Here's how the part is built. I have some questions about the finished solid (model axes, mm). Face numbers are marked on the shaded views. Coordinates: 2 decimals unless noted, no trailing zeros. Write each loop counter-clockwise with the first axis right and the second up, starting at its lowest first coordinate (ties: lowest second). Pieces come first, ordered by that corner, then holes. Notation, with made-up numbers: (75.5, 56) -> (96.5, 56) arc R14 cw to (96.5, 66) -> close; hole circle Ø7 at (44, 85). An arc over 180 degrees is marked (long way). Use a Markdown table: item, result. Add a question column.
Item 1: Imagine slicing it at A-A, the plane z = 2.85. Write out the boundary of the cut face in (x, y), and give its area (3 significant figures).
Item 2: Will these pins go through, and if not, where does the flat tip stop? pin 1 Ø1.5 at (y, z) = (-13, 1.5) entering from -X; pin 2 Ø1 at (x, y) = (10, -16.5) entering from +Z.
Item 3: If we mould it in two halves opening along Y, with no side actions, what happens to the marked faces 1 and 2? For each: pulls with the +Y half, pulls with the -Y half, needs draft (parallel to the pull), parting line crosses it, or undercut.
Item 4: If I drill on line 1 along Y through (x, z) = (0, 0.45); line 2 along Y through (x, z) = (0.5, 2.1); line 3 along X through (y, z) = (-7, 4.2), over which ranges is the centre line in solid material (lowest first)? Write a range as from..to.
```python
from build123d import *
from OCP.BRepFilletAPI import BRepFilletAPI_MakeChamfer

# Parameters (mm, degrees)
SKETCH_1_R          = 22
SKETCH_1_R_2        = 17.5
EXTRUDE_1_DEPTH     = 5
SKETCH_2_R          = 20.5
SKETCH_2_R_2        = 19
CUT_EXTRUDE_1_DEPTH = 0.5
CHAMFER_1_SIZE      = 0.2
CHAMFER_1_SIZE2     = 0.238350719
CHAMFER_2_SIZE      = 0.2
CHAMFER_2_SIZE2     = 0.238350719


with BuildPart() as part:
    # 草图1 → 凸台-拉伸1 (new body)
    with BuildSketch(Plane.XY):
        Circle(SKETCH_1_R)
        Circle(SKETCH_1_R_2, mode=Mode.SUBTRACT)
    extrude(amount=EXTRUDE_1_DEPTH)

    # 草图2 → 切除-拉伸1 (cut)
    with BuildSketch(Plane.XY.offset(5)):
        Circle(SKETCH_2_R)
        Circle(SKETCH_2_R_2, mode=Mode.SUBTRACT)
    cut_extrude_1 = extrude(amount=-CUT_EXTRUDE_1_DEPTH, mode=Mode.SUBTRACT)

    # 倒角1: one chamfer whose edges measure the first distance from different faces: ONE call of the kernel's chamfer builder (chamfer() names one face for all edges)
    chamfer_1_edges_1 = [part.edges().sort_by_distance(p)[0] for p in [
        (-20.5, 0, 4.5),
    ]]
    chamfer_1_side_1 = [part.faces().sort_by_distance(p)[0] for p in [
        (-20.5, 0, 4.75),
    ]]
    chamfer_1_edges_2 = [part.edges().sort_by_distance(p)[0] for p in [
        (-19, 0, 5),
    ]]
    chamfer_1_side_2 = [part.faces().sort_by_distance(p)[0] for p in [
        (-19, 0, 4.75),
    ]]
    chamfer_1_edges_3 = [part.edges().sort_by_distance(p)[0] for p in [
        (-22, 0, 5),
    ]]
    chamfer_1_side_3 = [part.faces().sort_by_distance(p)[0] for p in [
        (-22, 0, 2.5),
    ]]
    chamfer_1_edges_4 = [part.edges().sort_by_distance(p)[0] for p in [
        (-17.5, 0, 5),
    ]]
    chamfer_1_side_4 = [part.faces().sort_by_distance(p)[0] for p in [
        (-18.462598846, 0, 5),
    ]]
    chamfer_1 = BRepFilletAPI_MakeChamfer(part.part.solid().wrapped)
    for e in chamfer_1_edges_1:
        chamfer_1.Add(CHAMFER_1_SIZE, CHAMFER_1_SIZE2, e.wrapped, chamfer_1_side_1[0].wrapped)  # the first distance lies on this face
    for e in chamfer_1_edges_2:
        chamfer_1.Add(CHAMFER_1_SIZE, CHAMFER_1_SIZE2, e.wrapped, chamfer_1_side_2[0].wrapped)  # the first distance lies on this face
    for e in chamfer_1_edges_3:
        chamfer_1.Add(CHAMFER_1_SIZE, CHAMFER_1_SIZE2, e.wrapped, chamfer_1_side_3[0].wrapped)  # the first distance lies on this face
    for e in chamfer_1_edges_4:
        chamfer_1.Add(CHAMFER_1_SIZE, CHAMFER_1_SIZE2, e.wrapped, chamfer_1_side_4[0].wrapped)  # the first distance lies on this face
    add(Compound.cast(chamfer_1.Shape()), mode=Mode.REPLACE)

    # 镜向1: 切除-拉伸1 across plane
    add(cut_extrude_1.mirror(Plane.XY.offset(2.5)), mode=Mode.SUBTRACT)

    # 倒角2: one chamfer whose edges measure the first distance from different faces: ONE call of the kernel's chamfer builder (chamfer() names one face for all edges)
    chamfer_2_edges_1 = [part.edges().sort_by_distance(p)[0] for p in [
        (-22, 0, 0),
    ]]
    chamfer_2_side_1 = [part.faces().sort_by_distance(p)[0] for p in [
        (-21.377746033, 0, 0),
    ]]
    chamfer_2_edges_2 = [part.edges().sort_by_distance(p)[0] for p in [
        (-19, 0, 0),
    ]]
    chamfer_2_side_2 = [part.faces().sort_by_distance(p)[0] for p in [
        (-18.462598846, 0, 0),
    ]]
    chamfer_2_edges_3 = [part.edges().sort_by_distance(p)[0] for p in [
        (-20.5, 0, 0),
    ]]
    chamfer_2_side_3 = [part.faces().sort_by_distance(p)[0] for p in [
        (-20.5, 0, 0.25),
    ]]
    chamfer_2_edges_4 = [part.edges().sort_by_distance(p)[0] for p in [
        (-17.5, 0, 0),
    ]]
    chamfer_2_side_4 = [part.faces().sort_by_distance(p)[0] for p in [
        (-17.5, 0, 2.380824641),
    ]]
    chamfer_2 = BRepFilletAPI_MakeChamfer(part.part.solid().wrapped)
    for e in chamfer_2_edges_1:
        chamfer_2.Add(CHAMFER_2_SIZE, CHAMFER_2_SIZE2, e.wrapped, chamfer_2_side_1[0].wrapped)  # the first distance lies on this face
    for e in chamfer_2_edges_2:
        chamfer_2.Add(CHAMFER_2_SIZE, CHAMFER_2_SIZE2, e.wrapped, chamfer_2_side_2[0].wrapped)  # the first distance lies on this face
    for e in chamfer_2_edges_3:
        chamfer_2.Add(CHAMFER_2_SIZE, CHAMFER_2_SIZE2, e.wrapped, chamfer_2_side_3[0].wrapped)  # the first distance lies on this face
    for e in chamfer_2_edges_4:
        chamfer_2.Add(CHAMFER_2_SIZE, CHAMFER_2_SIZE2, e.wrapped, chamfer_2_side_4[0].wrapped)  # the first distance lies on this face
    add(Compound.cast(chamfer_2.Shape()), mode=Mode.REPLACE)


solid = part.part
```
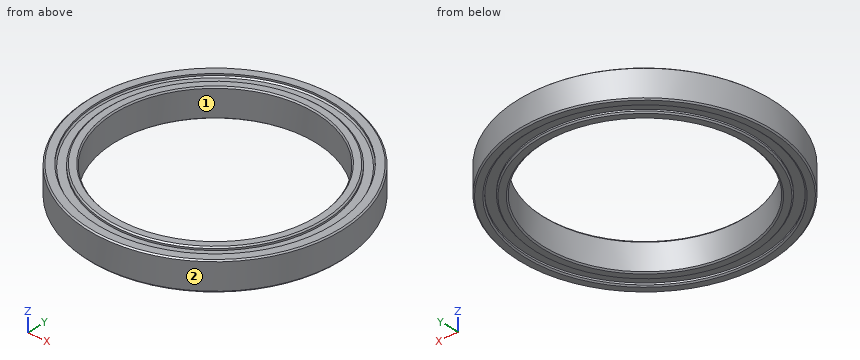
Ans:
| question | item | result |
|---|---|---|
| 1 | outline | circle Ø44 at (0, 0); hole circle Ø35 at (0, 0) |
| 1 | area | 558 mm^2 |
| 2 | pin 1 | stops at x = -18.27 |
| 2 | pin 2 | stops at z = 4.97 |
| 3 | face 1 | undercut |
| 3 | face 2 | parting line crosses it |
| 4 | line 1 | y = -22..-20.5, -19..-17.5, 17.5..19, 20.5..22 |
| 4 | line 2 | y = -21.99..-17.49, 17.49..21.99 |
| 4 | line 3 | x = -20.86..-16.04, 16.04..20.86 |
